from build123d import *

# Parameters (mm, degrees)
SKETCH1_R           = 1.5
SKETCH1_R_2         = 1.125
BOSS_EXTRUDE1_DEPTH = 5


with BuildPart() as part:
    # Sketch1 → Boss-Extrude1 (new body)
    with BuildSketch(Plane(origin=(0, 0, 0), x_dir=(1, 0, 0), z_dir=(0, 1, 0))):
        with BuildLine():
            Line((-38, -51), (38, -51))
            Line((38, -51), (38, -15))
            Line((38, -15), (48, -15))
            Line((48, -15), (48, 21))
            ThreePointArc((48, 21), (0, 45), (-48, 21))
            Line((-48, 21), (-48, -15))
            Line((-48, -15), (-38, -15))
            Line((-38, -15), (-38, -51))
        make_face()
        with Locations(Location((34, -48.04, 0), (0, 0, 270))):
            Circle(SKETCH1_R, mode=Mode.SUBTRACT)
        with Locations(Location((-34, -48.04, 0), (0, 0, 270))):
            Circle(SKETCH1_R, mode=Mode.SUBTRACT)
        with Locations(Location((-44, -11.04, 0), (0, 0, 270))):
            Circle(SKETCH1_R, mode=Mode.SUBTRACT)
        with Locations(Location((-44, 16.96, 0), (0, 0, 270))):
            Circle(SKETCH1_R, mode=Mode.SUBTRACT)
        with Locations(Location((44, 16.96, 0), (0, 0, 270))):
            Circle(SKETCH1_R, mode=Mode.SUBTRACT)
        with Locations(Location((44, -11.04, 0), (0, 0, 270))):
            Circle(SKETCH1_R, mode=Mode.SUBTRACT)
        with Locations(Location((-24, -26.24, 0), (0, 0, 270))):
            Circle(SKETCH1_R_2, mode=Mode.SUBTRACT)
        with Locations(Location((-24, -43.84, 0), (0, 0, 270))):
            Circle(SKETCH1_R_2, mode=Mode.SUBTRACT)
        with Locations(Location((24, -26.24, 0), (0, 0, 270))):
            Circle(SKETCH1_R_2, mode=Mode.SUBTRACT)
        with Locations(Location((24, -43.84, 0), (0, 0, 270))):
            Circle(SKETCH1_R_2, mode=Mode.SUBTRACT)
        with BuildLine():
            Line((-8, 28), (8, 28))
            Line((8, 28), (8, 21.5))
            Line((8, 21.5), (11, 21.5))
            ThreePointArc((11, 21.5), (12.5, 20), (11, 18.5))
            Line((11, 18.5), (8, 18.5))
            Line((8, 18.5), (8, 12))
            Line((8, 12), (-8, 12))
            Line((-8, 12), (-8, 18.5))
            Line((-8, 18.5), (-11, 18.5))
            ThreePointArc((-11, 18.5), (-12.5, 20), (-11, 21.5))
            Line((-11, 21.5), (-8, 21.5))
            Line((-8, 21.5), (-8, 28))
        make_face(mode=Mode.SUBTRACT)
    extrude(amount=BOSS_EXTRUDE1_DEPTH)


solid = part.part
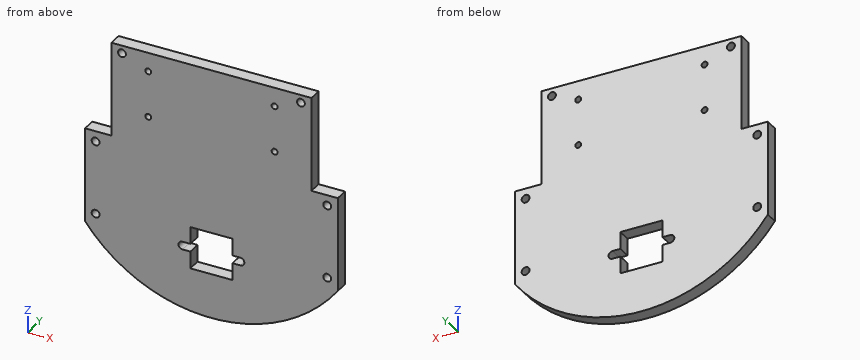
Design review of the part built by this model. Coordinates are the model's own, in mm. Give positions to 0.01 mm unless a question says otherwise; leave off trailing zeros. Loops run counter-clockwise (first coordinate to the right, second up) from the corner with the lowest first, then second, coordinate; pieces in that order, holes last. Notation, with made-up numbers: M 35,-21.5 L 40,-21.5 A24 ccw 40,-4.5 Z; hole C 60,-2 d9. An arc over 180 degrees is marked long. Answer as a JSON object with one key per item and string values.
Item 1: We need section D-D (x = -24). State the section outline as (y, z) points (3 decimals), and give its area (3 significant figures).
Output values:
{"outline": "M 0,-39.991 L 5,-39.991 L 5,25.115 L 0,25.115 Z; M 0,27.365 L 5,27.365 L 5,42.715 L 0,42.715 Z; M 0,44.965 L 5,44.965 L 5,51 L 0,51 Z", "area": "432 mm2"}
Item 2: We need section C-C (x = 1.5). State the section outline as (y, z) points.
Output values:
{"outline": "M 0,-44.98 L 5,-44.98 L 5,-28 L 0,-28 Z; M 0,-12 L 5,-12 L 5,51 L 0,51 Z"}
Item 3: For P1, Ø3.5, axis at x = 44, z = 11.04, coming from the +Y side; P2, Ø1, axis at x = -2.5, y = 1.5, coming from the -Z side; P3, Ø1.5, axis at x = -40.5, y = 3, coming from the +Z side; P4, Ø0.9, axis at x = 9, y = 1.5, coming from the -Z side, all flat-tipped, find the tip position at first contact; note any pin that passes through.
Output values:
{"P1": "stops at y = 5", "P2": "stops at z = -44.97", "P3": "stops at z = 15", "P4": "stops at z = -44.39"}
Item 4: We need section B-B (y = 3.1). Count the separate pieces of the cut face and the enclosed holes in it, and give its area (3 significant figures).
Output values:
{"separate pieces": "1", "enclosed holes": "11", "area": "7,460 mm2"}
Item 5: We need section A-A (z = 48.04). State the section outline as (x, y) points, and give its area (3 significant figures).
Output values:
{"outline": "M -38,0 L -35.5,0 L -35.5,5 L -38,5 Z; M -32.5,0 L 32.5,0 L 32.5,5 L -32.5,5 Z; M 35.5,0 L 38,0 L 38,5 L 35.5,5 Z", "area": "350 mm2"}
Item 6: Wall thickness on line 1 along X through (y, z) = (2.4, 43.84) (3 decimals); line 2 along X through (y, z) = (2.3, 11.04); line 3 along X through (y, z) = (3.4, -16.96): over which ranges is each line inside the solid? List them lowest first.
Output values:
{"line 1": "x = -38 to -25.125, -22.875 to 22.875, 25.125 to 38", "line 2": "x = -48 to -45.5, -42.5 to 42.5, 45.5 to 48", "line 3": "x = -48 to -45.5, -42.5 to -8, 8 to 42.5, 45.5 to 48"}
